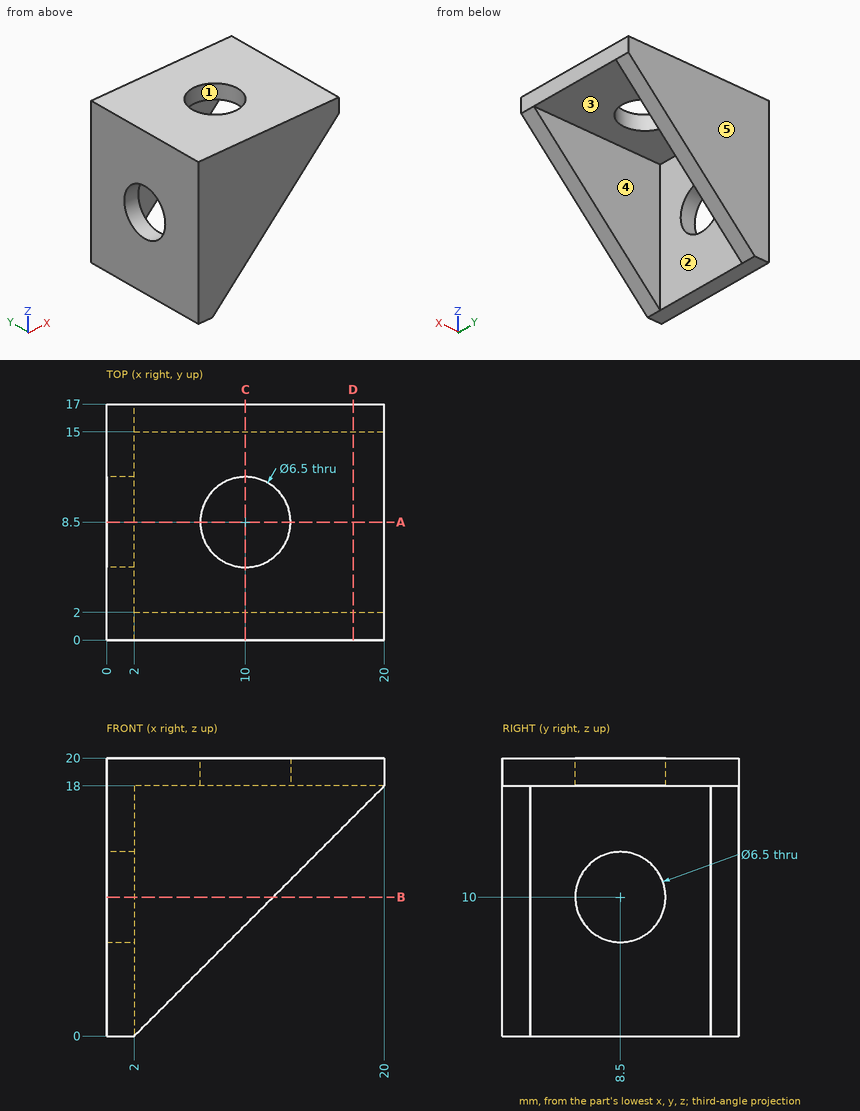
Input: dimensioned drawing with shaded views. Units: mm. Origin: part minimum x, y, z. A direction names the side the tool comes from. Coordinates: 2 decimals unless noted, no trailing zeros. Loops run counter-clockwise (first coordinate to the right, second up) from the corner with the lowest first, then second, coordinate; pieces in that order, holes last. Notation, with made-up numbers: (-36.5, 39) -> (-29.5, 39) arc R21 ccw to (-29.5, 55) -> close; hole circle Ø9 at (8, 44.5). An arc over 180 degrees is marked (long way). Use a Markdown table: item, result. Add a question column.
(1) Line query: line 1 along Y through (x, z) = (10, 18.5); line 2 along Y through (x, z) = (5, 13.5); line 3 along X through (y, z) = (8, 15.5). Output: solid intervals per line, ascending.
(2) Section query A-A, the plane y = 8.5. Return loops of the section in (x, z).
(3) Section query D-D, the plane x = 17.75. Return loops of the section in (y, z), plus the area to 3 significant figures.
(4) Section query C-C, the plane x = 10. Return loops of the section in (y, z), plus the area to 3 significant figures.
(5) Section query B-B, the plane z = 10. Return loops of the section in (x, y), plus the area to 3 significant figures.
(6) Access query for the marked faces 4 and 5. Directions: +Z, -Z, +X, -X, +Y, -Y. A direction counts if a zero-diameter tool reaches every point of the face in a straight line with its end or side. Return the directions, or none.
(7) Pin query (flat end, axial travel): pin 1 Ø5 at (x, y) = (15.5, 11.5) entering from -Z; pin 2 Ø5 at (y, z) = (7, 12.5) entering from -X; pin 3 Ø10 at (x, y) = (12, 14.5) entering from -Z. Return the tip coordinate at first contact, or that it passes through.
(8) Mould query, pull axis X, two halves, no side actions, for the marked faces 1, 2 and 3. Classes: pulls with the +X half, pulls with the -X half, needs draft (parallel to the pull), parting line crosses it, or undercut.
Answer:
| question | item | result |
|---|---|---|
| 1 | line 1 | y = 0 to 5.25, 11.75 to 17 |
| 1 | line 2 | y = 0 to 2, 15 to 17 |
| 1 | line 3 | x = 0 to 2 |
| 2 | outline | (0, 0) -> (2, 0) -> (2, 6.75) -> (0, 6.75) -> close; (0, 13.25) -> (2, 13.25) -> (2, 18) -> (6.75, 18) -> (6.75, 20) -> (0, 20) -> close; (13.25, 18) -> (20, 18) -> (20, 20) -> (13.25, 20) -> close |
| 3 | outline | (0, 15.75) -> (2, 15.75) -> (2, 18) -> (15, 18) -> (15, 15.75) -> (17, 15.75) -> (17, 20) -> (0, 20) -> close |
| 3 | area | 43.0 mm^2 |
| 4 | outline | (0, 8) -> (2, 8) -> (2, 18) -> (5.25, 18) -> (5.25, 20) -> (0, 20) -> close; (11.75, 18) -> (15, 18) -> (15, 8) -> (17, 8) -> (17, 20) -> (11.75, 20) -> close |
| 4 | area | 61.0 mm^2 |
| 5 | outline | (0, 0) -> (12, 0) -> (12, 2) -> (2, 2) -> (2, 5.25) -> (0, 5.25) -> close; (0, 11.75) -> (2, 11.75) -> (2, 15) -> (12, 15) -> (12, 17) -> (0, 17) -> close |
| 5 | area | 61.0 mm^2 |
| 6 | face 4 | -Z, +X |
| 6 | face 5 | +Z, -Z, +X, -X, +Y |
| 7 | pin 1 | stops at z = 18 |
| 7 | pin 2 | stops at x = 0 |
| 7 | pin 3 | stops at z = 5.03 |
| 8 | face 1 | undercut |
| 8 | face 2 | pulls with the +X half |
| 8 | face 3 | needs draft |
